```python
from build123d import *

# Parameters (mm, degrees)
SKETCH1_R           = 48
SKETCH1_R_2         = 44.5
BOSS_EXTRUDE3_DEPTH = 15
SKETCH1_5_R         = 48
SKETCH1_5_R_2       = 44.5
BOSS_EXTRUDE4_DEPTH = 2
FILLET1_R           = 1
CUT_EXTRUDE1_DEPTH  = 30
SKETCH4_R           = 2
CUT_EXTRUDE2_DEPTH  = 10


with BuildPart() as part:
    # Sketch1 → Boss-Extrude3 (new body)
    with BuildSketch(Plane(origin=(0, 0, 0), x_dir=(1, 0, 0), z_dir=(0, 1, 0))):
        Circle(SKETCH1_R)
        Circle(SKETCH1_R_2, mode=Mode.SUBTRACT)
    extrude(amount=-BOSS_EXTRUDE3_DEPTH)

    # Sketch1_5 → Boss-Extrude4 (add)
    with BuildSketch(Plane(origin=(0, 0, 0), x_dir=(1, 0, 0), z_dir=(0, 1, 0))):
        Circle(SKETCH1_5_R)
        Circle(SKETCH1_5_R_2, mode=Mode.SUBTRACT)
        Circle(SKETCH1_5_R_2)
    extrude(amount=BOSS_EXTRUDE4_DEPTH)

    # Fillet1
    fillet1_edges = [part.edges().sort_by_distance(p)[0] for p in [
        (-48, 2, 0),
        (-44.5, 0, 0),
    ]]
    fillet(fillet1_edges, radius=FILLET1_R)

    # Sketch3 → Cut-Extrude1 (cut)
    with BuildSketch(Plane(origin=(0, 2, 0), x_dir=(1, 0, 0), z_dir=(0, 1, 0))):
        Polygon((-29.45, 10), (-29.45, 0), (-29.45, -10), (10.55, -10), (10.55, 10), align=None)
    extrude(amount=-CUT_EXTRUDE1_DEPTH, mode=Mode.SUBTRACT)

    # Sketch4 → Cut-Extrude2 (cut)
    with BuildSketch(Plane(origin=(0, 2, 0), x_dir=(1, 0, 0), z_dir=(0, 1, 0))):
        with Locations((14.44886579, -5.09860841)):
            Circle(SKETCH4_R)
        with Locations((14.44886579, 5.09860841)):
            Circle(SKETCH4_R)
        with Locations((-33.34886579, -5.09860841)):
            Circle(SKETCH4_R)
        with Locations((-33.34886579, 5.09860841)):
            Circle(SKETCH4_R)
    extrude(amount=-CUT_EXTRUDE2_DEPTH, mode=Mode.SUBTRACT)


solid = part.part
```
The model under review builds one solid part; all positions refer to its coordinate system, in mm. A direction names the side the tool comes from. Round coordinates to 2 decimals unless told otherwise and drop trailing zeros. Order: outer loops, then holes, each group sorted by start corner. A loop starts at its lowest first (then second) coordinate and runs counter-clockwise, first axis right, second up.
(1) Take a section at C-C, the plane y = -3.25. State the section outline as (x, z) points, plus the area to 3 significant figures.
Working result:
outline: circle Ø96 at (0, 0); hole circle Ø89 at (0, 0)
area: 1,020 mm2
(2) Take a section at A-A, the plane z = 0. State the section outline as (x, y) points, plus the area to 3 significant figures.
Working result:
outline: (-48, -15) - (-44.5, -15) - (-44.5, -1) arc R1 cw to (-43.5, 0) - (-29.45, 0) - (-29.45, 2) - (-47, 2) arc R1 ccw to (-48, 1) - close; (10.55, 0) - (43.5, 0) arc R1 cw to (44.5, -1) - (44.5, -15) - (48, -15) - (48, 1) arc R1 ccw to (47, 2) - (10.55, 2) - close
area: 217 mm2
(3) Take a section at B-B, the plane x = 0. State the section outline as (y, z) points.
Working result:
outline: (-15, -48) - (1, -48) arc R1 ccw to (2, -47) - (2, -10) - (0, -10) - (0, -43.5) arc R1 cw to (-1, -44.5) - (-15, -44.5) - close; (-15, 44.5) - (-1, 44.5) arc R1 cw to (0, 43.5) - (0, 10) - (2, 10) - (2, 47) arc R1 ccw to (1, 48) - (-15, 48) - close
(4) Wall thickness on L1, parallel to Z at x = 0, y = -5.25; L2, parallel to Y at x = -34, z = 2; L3, parallel to Z at x = -10.5, y = -14: over which ranges is each line inside the solid? List them lowest first.
Working result:
L1: z = -48 to -44.5, 44.5 to 48
L2: y = 0 to 2
L3: z = -46.84 to -43.24, 43.24 to 46.84
(5) For P1, Ø0.6, axis at y = 1.5, z = 4.5, coming from the -X side; P2, Ø6, axis at x = 25.5, y = -3.5, coming from the +Z side; P3, Ø1.6, axis at x = -14.5, y = 1, coming from the -Z side; P4, Ø3.5, axis at x = 14.45, z = 5.1, coming from the +Y side, all flat-tipped, find the tip position at first contact; note any pin that passes through.
Working result:
P1: stops at x = -47.77
P2: stops at z = 42.4
P3: stops at z = -46
P4: passes through
(6) Mouldability with a two-part tool opening along X and no side actions: class faces 1 (the face through (14, -15, 42.4)), 2 (the face through (12.45, 1.01, 5.01)) as released by +X, released by -X, zero draft, split by the parting line, or undercut.
Working result:
face 1: zero draft
face 2: undercut
(7) Tool access review of faces 3 (the face through (-31.44, 1.01, 4.5)), 4 (the face through (-0.6, 0, -10.3)): name each direction out of +Z, -Z, +X, -X, +Y, -Y from which nothing blocks a thin tool from reaching the whole face with its end or side.
Working result:
face 3: +Y, -Y
face 4: -Y
